Verification items for the finished model (mm, model axes). A direction names the side the tool comes from. Coordinates: 2 decimals unless noted, no trailing zeros. Loops run counter-clockwise (first coordinate to the right, second up) from the corner with the lowest first, then second, coordinate; pieces in that order, holes last.
Q1. Sectioned sample at D-D (z = 12.7). Enter the section's corners in (x, y) (1 decimal), then the cut area to 3 significant figures.
Q2. Go/stop test with flat-tipped pins: P1, Ø1, axis at x = 9, y = 9, coming from the -Z side; P2, Ø11, axis at y = 14.5, z = -7, coming from the -X side; P3, Ø1, axis at x = 12, y = 18.5, coming from the +Z side; P4, Ø2.5, axis at x = 12.5, z = 11, coming from the +Y side. Record where each tip stops, or that it passes through.
Q3. Sectioned sample at C-C (y = 12). Enter the section's corners in (x, z).
Q4. Sectioned sample at B-B (x = 12.75). Enter the section's corners in (y, z) (3 decimals).
Q5. Sectioned sample at A-A (z = -5.08). Enter the section's corners in (x, y) (1 decimal).
Q6. Material ranges on probe 1 along Z at (x, y) = (12.25, 12.75); probe 2 along X at (y, z) = (1.25, -12.7); probe 3 along Y at (x, z) = (7.75, -5) (3 decimals), recorded low to high.
Q7. Access from +Z, -Z, +X, -X, +Y, -Y to the whole of each face (thin tool, end or side, straight path). Record for faces 4 (the face through (13, 15, 3.81)), 5 (the face through (0, 3.175, 0)), 6 (the face through (1, 0, 0)).
Q8. Mould release check, pull along X, two halves, no side actions. Record for faces 1 (the face through (13, 25.4, -8)), 2 (the face through (-0.344, 1.565, 10.18)), 3 (the face through (14.288, 10, -8)): +X half, -X half, draft (parallel to the pull), parting line (faces both ways), or undercut.
```python
from build123d import *

# Parameters (mm, degrees)
SKETCH1_W           = 22.225
SKETCH1_H           = 38.1
SKETCH1_R           = 3.175
BOSS_EXTRUDE1_DEPTH = 3.175
SKETCH2_W           = 3.175
SKETCH2_H           = 38.1
BOSS_EXTRUDE2_DEPTH = 25.4
SKETCH3_R           = 3.175
SKETCH3_W           = 15.24
SKETCH3_H           = 20.32
CUT_EXTRUDE1_DEPTH  = 39.75581408


with BuildPart() as part:
    # Sketch1 → Boss-Extrude1 (new body)
    with BuildSketch(Plane(origin=(0, 0, 0), x_dir=(1, 0, 0), z_dir=(0, 1, 0))):
        Rectangle(SKETCH1_W, SKETCH1_H)
        with Locations(Location((1.5875, 12.7, 0), (0, 0, 270))):
            Circle(SKETCH1_R, mode=Mode.SUBTRACT)
        with Locations(Location((1.5875, -12.7, 0), (0, 0, 270))):
            Circle(SKETCH1_R, mode=Mode.SUBTRACT)
    extrude(amount=BOSS_EXTRUDE1_DEPTH)

    # Sketch2 → Boss-Extrude2 (add)
    with BuildSketch(Plane(origin=(0, 0, 0), x_dir=(1, 0, 0), z_dir=(0, 1, 0))):
        with Locations((12.7, 0)):
            Rectangle(SKETCH2_W, SKETCH2_H)
    extrude(amount=BOSS_EXTRUDE2_DEPTH)

    # Sketch3 → Cut-Extrude1 (cut, through all)
    with BuildSketch(Plane.ZY.offset(-11.1125)):
        with Locations((-5.08, 12.7)):
            Circle(SKETCH3_R)
        with Locations((11.43, 15.24)):
            Rectangle(SKETCH3_W, SKETCH3_H)
    extrude(amount=-CUT_EXTRUDE1_DEPTH, mode=Mode.SUBTRACT)


solid = part.part
```
Geometry check:
1. outline: (-11.1, 0) - (-1.6, 0) - (-1.6, 3.2) - (-11.1, 3.2) - close; (4.8, 0) - (14.3, 0) - (14.3, 5.1) - (11.1, 5.1) - (11.1, 3.2) - (4.8, 3.2) - close
1. area: 66.5 mm2
2. P1: passes through
2. P2: stops at x = 11.11
2. P3: stops at z = 3.81
2. P4: stops at y = 5.08
3. outline: (11.11, -19.05) - (14.29, -19.05) - (14.29, -8.18) - (11.11, -8.18) - close; (11.11, -1.98) - (14.29, -1.98) - (14.29, 3.81) - (11.11, 3.81) - close
4. outline: (0, -19.05) - (25.4, -19.05) - (25.4, 3.81) - (5.08, 3.81) - (5.08, 19.05) - (0, 19.05) - close; hole circle Ø6.35 at (12.7, -5.08)
5. outline: (-11.1, 0) - (14.3, 0) - (14.3, 9.5) - (11.1, 9.5) - (11.1, 3.2) - (-11.1, 3.2) - close; (11.1, 15.9) - (14.3, 15.9) - (14.3, 25.4) - (11.1, 25.4) - close
6. probe 1: z = -19.05 to -8.25, -1.91 to 3.81
6. probe 2: x = -11.11 to -1.59, 4.76 to 14.29
6. probe 3: y = 0 to 3.175
7. face 4: +Z, +X, -X, +Y
7. face 5: +Z, -Z, -X, +Y
7. face 6: +Z, -Z, +X, -X, -Y
8. face 1: draft
8. face 2: undercut
8. face 3: +X half
